Here's how the part is built. I have some questions about the finished solid (model axes, mm). Face numbers are marked on the shaded views. Give positions to 0.01 mm unless a question says otherwise; leave off trailing zeros. Order: outer loops, then holes, each group sorted by start corner. A loop starts at its lowest first (then second) coordinate and runs counter-clockwise, first axis right, second up. Notation, with made-up numbers: M 11,13 L 51,13 A19 ccw 51,27 Z; hole C -39.5,-34 d8. An arc over 180 degrees is marked long. Use one line per item in the form item = value.
from build123d import *

# Parameters (mm, degrees)
SKETCH1_W           = 27.94
SKETCH1_H           = 23.114
BOSS_EXTRUDE1_DEPTH = 12.954
SKETCH2_R           = 5.05
CUT_EXTRUDE1_DEPTH  = 13.954
SKETCH3_W           = 13.97
SKETCH3_H           = 1.524
CUT_EXTRUDE2_DEPTH  = 13.954
SKETCH4_R           = 1.25
CUT_EXTRUDE3_DEPTH  = 13.954
SKETCH5_R           = 3.048
CUT_EXTRUDE4_DEPTH  = 4.318
CUT_EXTRUDE5_REACH  = 20.796
SKETCH6_R           = 1.7
SKETCH7_R           = 1.25
CUT_EXTRUDE6_DEPTH  = 19.796


with BuildPart() as part:
    # Sketch1 → Boss-Extrude1 (new body)
    with BuildSketch(Plane(origin=(0, 0, 0), x_dir=(1, 0, 0), z_dir=(0, 1, 0))):
        Rectangle(SKETCH1_W, SKETCH1_H)
    extrude(amount=BOSS_EXTRUDE1_DEPTH)

    # Sketch2 → Cut-Extrude1 (cut, through all)
    with BuildSketch(Plane(origin=(0, 12.954, 0), x_dir=(1, 0, 0), z_dir=(0, 1, 0))):
        with Locations((0, 2.667)):
            Circle(SKETCH2_R)
    extrude(amount=-CUT_EXTRUDE1_DEPTH, mode=Mode.SUBTRACT)

    # Sketch3 → Cut-Extrude2 (cut, through all)
    with BuildSketch(Plane(origin=(0, 12.954, 0), x_dir=(1, 0, 0), z_dir=(0, 1, 0))):
        with Locations((6.985, 2.667)):
            Rectangle(SKETCH3_W, SKETCH3_H)
    extrude(amount=-CUT_EXTRUDE2_DEPTH, mode=Mode.SUBTRACT)

    # Sketch4 → Cut-Extrude3 (cut, through all)
    with BuildSketch(Plane(origin=(0, 12.954, 0), x_dir=(1, 0, 0), z_dir=(0, 1, 0))):
        with Locations((-9.906, 8.509)):
            Circle(SKETCH4_R)
        with Locations((5.08, -7.493)):
            Circle(SKETCH4_R)
    extrude(amount=-CUT_EXTRUDE3_DEPTH, mode=Mode.SUBTRACT)

    # Sketch5 → Cut-Extrude4 (cut)
    with BuildSketch(Plane(origin=(0, 0, -11.557), x_dir=(-1, 0, 0), z_dir=(0, 0, -1))):
        with Locations((-9.906, 6.35)):
            Circle(SKETCH5_R)
    extrude(amount=-CUT_EXTRUDE4_DEPTH, mode=Mode.SUBTRACT)

    # Sketch6 → Cut-Extrude5 (cut, up to next)
    with BuildSketch(Plane(origin=(0, 0, -7.239), x_dir=(-1, 0, 0), z_dir=(0, 0, -1)), mode=Mode.PRIVATE) as cut_extrude5_sk1:
        with Locations((-9.906, 6.35)):
            Circle(SKETCH6_R)
    cut_extrude5_tool1 = extrude(cut_extrude5_sk1.sketch, amount=-CUT_EXTRUDE5_REACH, mode=Mode.PRIVATE) & part.part
    add(cut_extrude5_tool1.solids().sort_by_distance((9.906, 6.35, -7.239))[0], mode=Mode.SUBTRACT)

    # Sketch7 → Cut-Extrude6 (cut, through all)
    with BuildSketch(Plane(origin=(0, 0, -7.239), x_dir=(-1, 0, 0), z_dir=(0, 0, -1))):
        with Locations((-9.906, 6.35)):
            Circle(SKETCH7_R)
    extrude(amount=-CUT_EXTRUDE6_DEPTH, mode=Mode.SUBTRACT)


solid = part.part
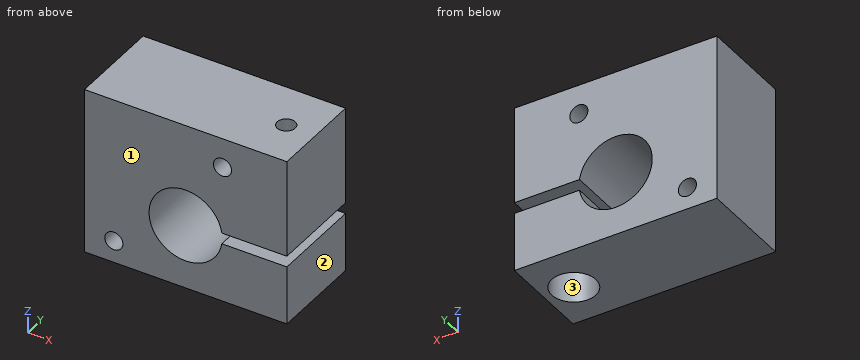
Q1. I want a section at A-A on z = -0.5. Write out the boundary of the cut face in (x, y), then the cut area to 3 significant figures.
Found:
outline = M -13.97,0 L -4.56,0 L -4.56,12.95 L -13.97,12.95 Z; M 4.56,0 L 13.97,0 L 13.97,12.95 L 4.56,12.95 Z; hole C 9.91,6.35 d2.5
area = 239 mm²
Q2. I need wall thicknesses on L1, parallel to Z at x = 5.08, y = 4 (3 decimals); L2, parallel to Z at x = 0, y = 8.25; L3, parallel to Z at x = 5.5, y = 7.5 (3 decimals). Which ranges of each line are inside material? Lowest first, please.
Found:
L1 = -11.557 to -3.429, -1.905 to 6.243, 8.743 to 11.557
L2 = -11.56 to -7.72, 2.38 to 11.56
L3 = -11.557 to -3.429, -1.905 to 6.316, 8.67 to 11.557
Q3. Thinking about a two-plate mould opening in Y: for the marked faces 1, 2 and 3, which applies, +Y half, -Y half, draft (parallel to the pull), parting line (faces both ways), or undercut?
Found:
face_1 = -Y half
face_2 = draft
face_3 = undercut
Q4. I want a section at D-D on y = 3.75. Write out the boundary of the cut face in (x, z) (3 decimals).
Found:
outline = M -13.97,-11.557 L 8.315,-11.557 L 8.315,-7.239 L 11.497,-7.239 L 11.497,-11.557 L 13.97,-11.557 L 13.97,-3.429 L 4.992,-3.429 A5.05 cw long 4.992,-1.905 L 13.97,-1.905 L 13.97,11.557 L -13.97,11.557 Z; hole C -9.906,-8.509 d2.5; hole C 5.08,7.493 d2.5
Q5. I want a section at C-C on x = 6. Write out the boundary of the cut face in (y, z) (3 decimals).
Found:
outline = M 0,-11.557 L 12.954,-11.557 L 12.954,-3.429 L 0,-3.429 Z; M 0,-1.905 L 12.954,-1.905 L 12.954,6.647 L 0,6.647 Z; M 0,8.339 L 12.954,8.339 L 12.954,11.557 L 0,11.557 Z
Q6. I want a section at B-B on x = 0. Write out the boundary of the cut face in (y, z).
Found:
outline = M 0,-11.56 L 12.95,-11.56 L 12.95,-7.72 L 0,-7.72 Z; M 0,2.38 L 12.95,2.38 L 12.95,11.56 L 0,11.56 Z
Q7. I'm going to push flat-ended pins straight in: pin 1 Ø6 at (x, z) = (0, -2.667) entering from -Y; pin 2 Ø2.5 at (x, y) = (11, 5.5) entering from -Z; pin 3 Ø3 at (x, y) = (9.906, 6.35) entering from -Z (3 decimals). Where does each tip first touch, or does it pass through?
Found:
pin_1 = through
pin_2 = -7.24
pin_3 = -1.905
